from build123d import *

# Parameters (mm, degrees)
PAD_DEPTH       = 6
SKETCH002_W     = 7.4
SKETCH002_H     = 66
SKETCH002_W_2   = 18
SKETCH002_H_2   = 7.4
PAD001_DEPTH    = 0.4
SKETCH003_R     = 1.6
POCKET_DEPTH    = 6.401
SKETCH004_R     = 3
POCKET001_DEPTH = 1
SKETCH005_R     = 4
PAD002_DEPTH    = 0.2
CHAMFER_SIZE    = 0.4
FILLET_R        = 2


with BuildPart() as part:
    # Sketch → Pad (new body)
    with BuildSketch(Plane.XY):
        Polygon((-9.75, 34), (-9.75, -34), (29.25, -34), (29.25, -15), (9.75, -15), (9.75, 15), (29.25, 15), (29.25, 34), (9.75, 34), align=None)
    extrude(amount=PAD_DEPTH)

    # Sketch002 → Pad001 (new body)
    with BuildSketch(Plane.XY.offset(6)):
        Rectangle(SKETCH002_W, SKETCH002_H)
        with Locations((19.25, 24.5)):
            Rectangle(SKETCH002_W_2, SKETCH002_H_2)
        with Locations((19.25, -24.5)):
            Rectangle(SKETCH002_W_2, SKETCH002_H_2)
    extrude(amount=PAD001_DEPTH)

    # Sketch003 → Pocket (cut, through all)
    with BuildSketch(Plane(origin=(0, 0, 0), x_dir=(1, 0, 0), z_dir=(0, 0, -1))):
        with Locations((0, 24.5)):
            Circle(SKETCH003_R)
        with Locations((19.5, 24.5)):
            Circle(SKETCH003_R)
        with Locations((0, -24.5)):
            Circle(SKETCH003_R)
        with Locations((19.5, -24.5)):
            Circle(SKETCH003_R)
    extrude(amount=-POCKET_DEPTH, mode=Mode.SUBTRACT)

    # Sketch004 → Pocket001 (cut)
    with BuildSketch(Plane(origin=(0, 0, 0), x_dir=(1, 0, 0), z_dir=(0, 0, -1))):
        with Locations((0, 24.5)):
            Circle(SKETCH004_R)
        with Locations((19.5, 24.5)):
            Circle(SKETCH004_R)
        with Locations((0, -24.5)):
            Circle(SKETCH004_R)
        with Locations((19.5, -24.5)):
            Circle(SKETCH004_R)
    extrude(amount=-POCKET001_DEPTH, mode=Mode.SUBTRACT)

    # Sketch005 → Pad002 (new body)
    with BuildSketch(Plane(origin=(0, 0, 1), x_dir=(1, 0, 0), z_dir=(0, 0, -1))):
        with Locations((0, 24.5)):
            Circle(SKETCH005_R)
        with Locations((19.5, 24.5)):
            Circle(SKETCH005_R)
        with Locations((0, -24.5)):
            Circle(SKETCH005_R)
        with Locations((19.5, -24.5)):
            Circle(SKETCH005_R)
    extrude(amount=-PAD002_DEPTH)

    # Chamfer
    chamfer_edges = [part.edges().sort_by_distance(p)[0] for p in [
        (16.5, -24.5, 0),
        (16.5, 24.5, 0),
        (-3, -24.5, 0),
        (-3, 24.5, 0),
    ]]
    chamfer(chamfer_edges, length=CHAMFER_SIZE)

    # Fillet
    fillet_edges = [part.edges().sort_by_distance(p)[0] for p in [
        (9.75, 15, 3),
        (9.75, 0, 0),
        (19.5, 15, 0),
        (9.75, -15, 3),
        (19.5, -15, 0),
        (29.25, -15, 3),
        (29.25, 15, 3),
        (29.25, 24.5, 0),
        (29.25, -24.5, 0),
        (29.25, -34, 3),
        (9.75, -34, 0),
        (29.25, 34, 3),
        (9.75, 34, 0),
        (-9.75, 34, 3),
        (-9.75, 0, 0),
        (-9.75, -34, 3),
    ]]
    fillet(fillet_edges, radius=FILLET_R)


solid = part.part
Geometry: final body of the model. Coordinates: model frame, mm. A direction names the side the tool comes from. Round coordinates to 2 decimals unless told otherwise and drop trailing zeros. Write each loop counter-clockwise with the first axis right and the second up, starting at its lowest first coordinate (ties: lowest second). Pieces come first, ordered by that corner, then holes. Notation, with made-up numbers: M 35.25,-37.5 L 77.25,-37.5 A19 cw 77.25,-33.5 Z; hole C 26,4 d1. An arc over 180 degrees is marked long. Write item = value, one per line.
Item 1: Pull-direction query (X, two-part tool) for faces 6 (the face through (0, 24, 1)), 7 (the face through (9.5, 33.4, 0.57)), 8 (the face through (10.35, 14.43, 4.03)); classes: pulls with the +X half, pulls with the -X half, needs draft (parallel to the pull), parting line crosses it, or undercut.
Findings:
face_6 = undercut
face_7 = needs draft
face_8 = pulls with the +X half
Item 2: Section query A-A on x = 25.5. Return loops of the section in (y, z).
Findings:
outline = M -34,2 A2 ccw -32,0 L -17,0 A2 ccw -15,2 L -15,6 L -20.8,6 L -20.8,6.4 L -28.2,6.4 L -28.2,6 L -34,6 Z; M 15,2 A2 ccw 17,0 L 32,0 A2 ccw 34,2 L 34,6 L 28.2,6 L 28.2,6.4 L 20.8,6.4 L 20.8,6 L 15,6 Z
Item 3: Material intervals for line 1 along X through (y, z) = (24.5, 3.95); line 2 along Y through (x, z) = (19.5, 5); line 3 along Y through (x, z) = (0, 4.15), sorted ascending. Write a range as [from, to].
Findings:
line_1 = [-9.75, -1.6], [1.6, 17.9], [21.1, 29.25]
line_2 = [-34, -26.1], [-22.9, -15], [15, 22.9], [26.1, 34]
line_3 = [-34, -26.1], [-22.9, 22.9], [26.1, 34]
Item 4: Section query B-B on y = 3. Return loops of the section in (x, z), then the cut area to 3 significant figures.
Findings:
outline = M -9.75,2 A2 ccw -7.75,0 L 7.75,0 A2 ccw 9.75,2 L 9.75,6 L 3.7,6 L 3.7,6.4 L -3.7,6.4 L -3.7,6 L -9.75,6 Z
area = 118 mm^2
Item 5: Access query for faces 1 (the face through (29.25, 24, 4)), 2 (the face through (0, 24, 1.2)), 3 (the face through (0, -25, 1)), 4 (the face through (28.65, 24.6, 0.57)), 5 (the face through (19.61, 15.6, 0.57)). Directions: +Z, -Z, +X, -X, +Y, -Y. A direction counts if a zero-diameter tool reaches every point of the face in a straight line with its end or side. Return the directions, or none.
Findings:
face_1 = +Z, -Z, +X, +Y, -Y
face_2 = +Z
face_3 = -Z
face_4 = -Z, +X, +Y, -Y
face_5 = -Z, +X
Item 6: Section query C-C on z = 2.75. Return loops of the section in (x, y), then the cut area to 3 significant figures.
Findings:
outline = M -9.75,-32 A2 ccw -7.75,-34 L 27.25,-34 A2 ccw 29.25,-32 L 29.25,-17 A2 ccw 27.25,-15 L 11.75,-15 A2 cw 9.75,-13 L 9.75,13 A2 cw 11.75,15 L 27.25,15 A2 ccw 29.25,17 L 29.25,32 A2 ccw 27.25,34 L -7.75,34 A2 ccw -9.75,32 Z; hole C 0,-24.5 d3.2; hole C 0,24.5 d3.2; hole C 19.5,-24.5 d3.2; hole C 19.5,24.5 d3.2
area = 2,030 mm^2
Item 7: Pin query (flat end, axial travel): P1, Ø1.9, axis at x = 0, y = -24.5, coming from the -Z side; P2, Ø1.5, axis at x = 6, y = -14.5, coming from the +Z side; P3, Ø1.6, axis at x = 19.5, y = 24, coming from the +Z side. Return the tip coordinate at first contact, or that it passes through.
Findings:
P1 = 1
P2 = 6
P3 = 1.2
